Print and shaded views of the part. All mm, measured from the part's lowest x, y and z. Give positions to 0.01 mm unless a question says otherwise; leave off trailing zeros. Loops run counter-clockwise (first coordinate to the right, second up) from the corner with the lowest first, then second, coordinate; pieces in that order, holes last. Notation, with made-up numbers: M 7,49.25 L 40,49.25 A14 ccw 40,61.25 Z; hole C 30,68.5 d8. An arc over 180 degrees is marked long. Answer as CSV lines item,"result".
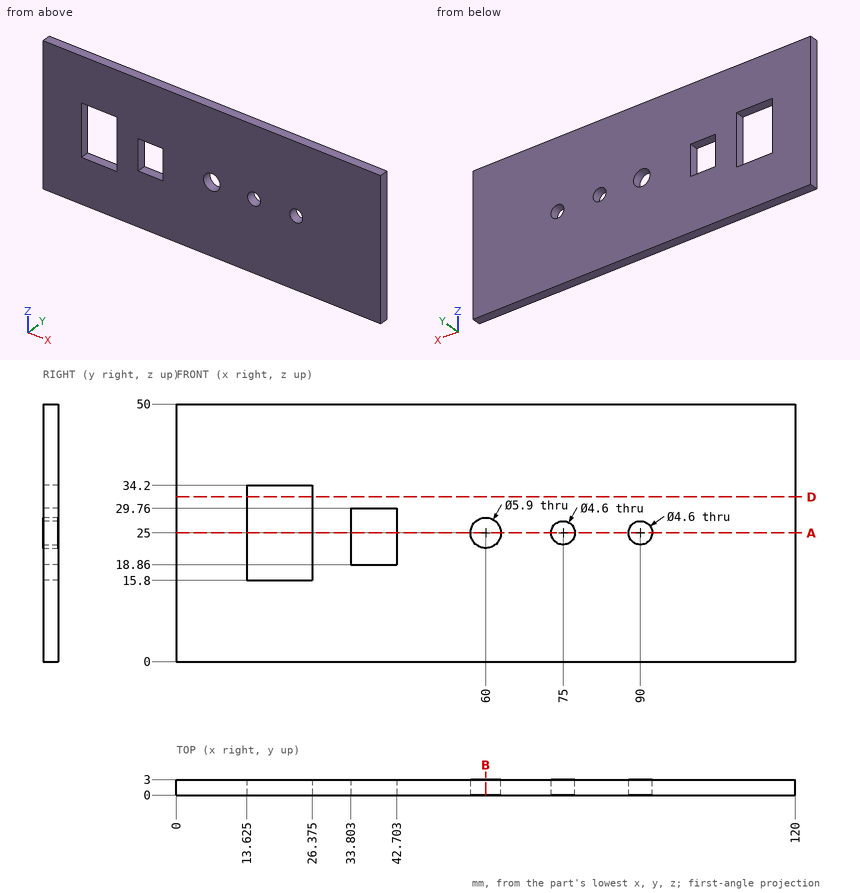
Q1. Cut at B-B (x = 60). Write the cut outline in (y, z).
Solution:
outline,"M 0,0 L 3,0 L 3,22.05 L 0,22.05 Z; M 0,27.95 L 3,27.95 L 3,50 L 0,50 Z"
Q2. Wall check: line 1 (X direction, y = 1.2, z = 22) (1 decimal); line 2 (Z direction, x = 23, y = 0.5); line 3 (Z direction, x = 42, y = 1). Give the ranges that are in metal, low to high. Write a range as [from, to].
Solution:
line 1,"x = [0, 13.6], [26.4, 33.8], [42.7, 120]"
line 2,"z = [0, 15.8], [34.2, 50]"
line 3,"z = [0, 18.86], [29.76, 50]"
Q3. Cut at A-A (z = 25). Give the number of separate pieces and of enclosed holes in the cut face, and give its area (3 significant figures).
Solution:
separate pieces,"6"
enclosed holes,"0"
area,"250 mm²"
Q4. Pin check, flat tip, straight feed: P1, Ø1.5, axis at x = 17.5, y = 1.5, coming from the -Z side. Stop position of the tip, or through.
Solution:
P1,"stops at z = 0"
Q5. Cut at D-D (z = 32). Write the cut outline in (x, y) (1 decimal).
Solution:
outline,"M 0,0 L 13.6,0 L 13.6,3 L 0,3 Z; M 26.4,0 L 120,0 L 120,3 L 26.4,3 Z"
